Work out the finished part from the listing and answer in its coordinate system (mm). Give positions to 0.01 mm unless a question says otherwise; leave off trailing zeros. Order: outer loops, then holes, each group sorted by start corner. A loop starts at its lowest first (then second) coordinate and runs counter-clockwise, first axis right, second up. Notation, with made-up numbers: (-19, 50) -> (6, 50) arc R33 ccw to (6, 88) -> close; hole circle Ø4 at (52.25, -32.5). An arc over 180 degrees is marked (long way). Use a Markdown table: item, result. Add a question column.
```python
from build123d import *

# Parameters (mm, degrees)
SKETCH1_R           = 1.7
BOSS_EXTRUDE1_DEPTH = 1.5
FILLET1_R           = 5


with BuildPart() as part:
    # Sketch1 → Boss-Extrude1 (new body)
    with BuildSketch(Plane(origin=(0, 0, 0), x_dir=(1, 0, 0), z_dir=(0, 1, 0))):
        Polygon((-12.939466701, 37.882793222), (-12.939466701, -47.467206778), (52.550533299, -47.467206778), (52.550533299, 37.882793222), (29.080533299, 37.882793222), (29.080533299, 6.882793222), (10.580533299, 6.882793222), (10.580533299, 37.882793222), align=None)
        with Locations(Location((-7.939466701, -42.467206778, 0), (0, 0, 270))):
            Circle(SKETCH1_R, mode=Mode.SUBTRACT)
        with BuildLine():
            ThreePointArc((2.241533299, -19.596771318), (2.37153922, -19.282909259), (2.685401279, -19.152903338))
            Line((2.685401279, -19.152903338), (14.22596876, -19.152903338))
            ThreePointArc((14.22596876, -19.152903338), (14.539830818, -19.282909259), (14.66983674, -19.596771318))
            Line((14.66983674, -19.596771318), (14.66983674, -31.137338798))
            ThreePointArc((14.66983674, -31.137338798), (14.539830818, -31.451200857), (14.22596876, -31.581206778))
            Line((14.22596876, -31.581206778), (2.685401279, -31.581206778))
            ThreePointArc((2.685401279, -31.581206778), (2.37153922, -31.451200857), (2.241533299, -31.137338798))
            Line((2.241533299, -31.137338798), (2.241533299, -19.596771318))
        make_face(mode=Mode.SUBTRACT)
        with BuildLine():
            ThreePointArc((2.241533299, -2.685401279), (2.37153922, -2.37153922), (2.685401279, -2.241533299))
            Line((2.685401279, -2.241533299), (14.22596876, -2.241533299))
            ThreePointArc((14.22596876, -2.241533299), (14.539830818, -2.37153922), (14.66983674, -2.685401279))
            Line((14.66983674, -2.685401279), (14.66983674, -14.22596876))
            ThreePointArc((14.66983674, -14.22596876), (14.539830818, -14.539830818), (14.22596876, -14.66983674))
            Line((14.22596876, -14.66983674), (2.685401279, -14.66983674))
            ThreePointArc((2.685401279, -14.66983674), (2.37153922, -14.539830818), (2.241533299, -14.22596876))
            Line((2.241533299, -14.22596876), (2.241533299, -2.685401279))
        make_face(mode=Mode.SUBTRACT)
        with Locations(Location((47.550533299, -42.467206778, 0), (0, 0, 270))):
            Circle(SKETCH1_R, mode=Mode.SUBTRACT)
        with BuildLine():
            ThreePointArc((19.152903338, -19.596771318), (19.282909259, -19.282909259), (19.596771318, -19.152903338))
            Line((19.596771318, -19.152903338), (31.137338798, -19.152903338))
            ThreePointArc((31.137338798, -19.152903338), (31.451200857, -19.282909259), (31.581206778, -19.596771318))
            Line((31.581206778, -19.596771318), (31.581206778, -31.137338798))
            ThreePointArc((31.581206778, -31.137338798), (31.451200857, -31.451200857), (31.137338798, -31.581206778))
            Line((31.137338798, -31.581206778), (19.596771318, -31.581206778))
            ThreePointArc((19.596771318, -31.581206778), (19.282909259, -31.451200857), (19.152903338, -31.137338798))
            Line((19.152903338, -31.137338798), (19.152903338, -19.596771318))
        make_face(mode=Mode.SUBTRACT)
        with BuildLine():
            ThreePointArc((19.152903338, -2.685401279), (19.282909259, -2.37153922), (19.596771318, -2.241533299))
            Line((19.596771318, -2.241533299), (31.137338798, -2.241533299))
            ThreePointArc((31.137338798, -2.241533299), (31.451200857, -2.37153922), (31.581206778, -2.685401279))
            Line((31.581206778, -2.685401279), (31.581206778, -14.22596876))
            ThreePointArc((31.581206778, -14.22596876), (31.451200857, -14.539830818), (31.137338798, -14.66983674))
            Line((31.137338798, -14.66983674), (19.596771318, -14.66983674))
            ThreePointArc((19.596771318, -14.66983674), (19.282909259, -14.539830818), (19.152903338, -14.22596876))
            Line((19.152903338, -14.22596876), (19.152903338, -2.685401279))
        make_face(mode=Mode.SUBTRACT)
        with Locations(Location((-7.939466701, 32.882793222, 0), (0, 0, 270))):
            Circle(SKETCH1_R, mode=Mode.SUBTRACT)
        with Locations(Location((47.550533299, 32.882793222, 0), (0, 0, 270))):
            Circle(SKETCH1_R, mode=Mode.SUBTRACT)
    extrude(amount=BOSS_EXTRUDE1_DEPTH)

    # Fillet1
    fillet1_edges = [part.edges().sort_by_distance(p)[0] for p in [
        (52.550533299, 0.75, -37.882793222),
        (52.550533299, 0.75, 47.467206778),
        (-12.939466701, 0.75, 47.467206778),
        (-12.939466701, 0.75, -37.882793222),
    ]]
    fillet(fillet1_edges, radius=FILLET1_R)


solid = part.part
```
1) The part is cut by section D-D, the plane y = 1.05. State how many separate pieces and enclosed holes the cut face has, then the cut area to 3 significant figures.
2) The part is cut by section C-C, the plane z = 24.5. Determine the outline of the cut face in (x, y).
3) Straight lines are drawn through the part: line 1 (X direction, y = 0.9, z = 8.5); line 2 (Z direction, x = 28.5, y = 0.1); line 3 (Z direction, x = 5.5, y = 1). For each, find the intervals that lie inside material, in ascending order.
4) The part is cut by section B-B, the plane z = -11.5. Determine the outline of the cut face in (x, y).
5) Flat-ended cylindrical pins translate along their axes: pin 1 (0.8 mm diameter, centred on x = 15.5, y = 0.5, fed in from -Z); pin 2 (2 mm diameter, centred on x = 1, z = 27.5, fed in from -Y); pin 3 (2.5 mm diameter, centred on x = 47.55, z = 42.47, fed in from +Y). Find the tip coordinate at first contact, or state that the pin passes through.
6) The part is cut by section A-A, the plane x = 9. Determine the outline of the cut face in (y, z).
A:
| question | item | result |
|---|---|---|
| 1 | separate pieces | 1 |
| 1 | enclosed holes | 8 |
| 1 | area | 4,340 mm^2 |
| 2 | outline | (-12.94, 0) -> (2.24, 0) -> (2.24, 1.5) -> (-12.94, 1.5) -> close; (14.67, 0) -> (19.15, 0) -> (19.15, 1.5) -> (14.67, 1.5) -> close; (31.58, 0) -> (52.55, 0) -> (52.55, 1.5) -> (31.58, 1.5) -> close |
| 3 | line 1 | -12.94 to 2.24, 14.67 to 19.15, 31.58 to 52.55 |
| 3 | line 2 | -6.88 to 2.24, 14.67 to 19.15, 31.58 to 47.47 |
| 3 | line 3 | -37.88 to 2.24, 14.67 to 19.15, 31.58 to 47.47 |
| 4 | outline | (-12.94, 0) -> (10.58, 0) -> (10.58, 1.5) -> (-12.94, 1.5) -> close; (29.08, 0) -> (52.55, 0) -> (52.55, 1.5) -> (29.08, 1.5) -> close |
| 5 | pin 1 | z = -6.88 |
| 5 | pin 2 | y = 0 |
| 5 | pin 3 | through |
| 6 | outline | (0, -37.88) -> (1.5, -37.88) -> (1.5, 2.24) -> (0, 2.24) -> close; (0, 14.67) -> (1.5, 14.67) -> (1.5, 19.15) -> (0, 19.15) -> close; (0, 31.58) -> (1.5, 31.58) -> (1.5, 47.47) -> (0, 47.47) -> close |
